Source: CAD feature listing. Evaluate the final solid. Frame: model axes, mm. A direction names the side the tool comes from. Coordinates: 2 decimals unless noted, no trailing zeros. Loops run counter-clockwise (first coordinate to the right, second up) from the corner with the lowest first, then second, coordinate; pieces in that order, holes last.
Item 1: Section query A-A, the plane y = 0. Return the cut outline in (x, z), then the cut area to 3 significant figures.
Item 2: Section query B-B, the plane x = -79.5. Return the cut outline in (y, z).
Item 3: Pin query (flat end, axial travel): pin 1 Ø3 at (x, z) = (-99.5, 72.5) entering from +Y; pin 2 Ø8 at (y, z) = (-39.5, 93) entering from +X; pin 3 Ø6 at (x, z) = (-19.5, 170) entering from +Y. Return the tip coordinate at first contact, or that it passes through.
Item 4: Section query D-D, the plane y = 279. Return the cut outline in (x, z).
Item 5: Line query: probe 1 along Y at (x, z) = (0, 71); probe 2 along Z at (x, y) = (103.5, 95.5); probe 3 along Z at (x, y) = (82, 193). Output: solid intervals per line, ascending.
Item 6: Reachability of faces 1 (the flat face through (100, 210, 188)), 2 (the cylindrical face through (-19.527, 148.724, -7.395)), 3 (the cylindrical face through (123.997, -39.048, 88.74)) from +Z, -Z, +X, -X, +Y, -Y: full face, straight path, thin tool, end or side. Return the list, or none.
Item 7: Pull-direction query (X, two-part tool) for faces 4 (the flat face through (1, 311.803, 188)), 5 (the flat face through (-100, 213, 188)), 6 (the cylindrical face through (-30.04, -95.38, 88.53)); classes: +X half, -X half, draft (parallel to the pull), parting line (faces both ways), or undercut.
Item 8: Section query C-C, the plane z = 68.5. Return the cut outline in (x, y).
Autodesk Inventor part; units mm, degrees
ref_plane "Work Plane3" through (0, 0, 90) normal (0, 0, -1) x (-1, 0, 0)
ref_plane "YZ Plane" through (0, 0, 0) normal (1, 0, 0) x (0, 1, 0)
ref_plane "XZ Plane" through (0, 0, 0) normal (0, 1, 0) x (-1, 0, 0)
sketch "Sketch1" plane through (0, 0, 0) normal (0, 0, 1) x (1, 0, 0)
  circle A0 centre (0, 0) radius 130
  dimension "d0" = 260
extrude "Extrusion1" add sketch "Sketch1" along normal blind 180
sketch "Sketch2" plane through (0, 0, 180) normal (0, 0, 1) x (1, 0, 0)
  circle A0 centre (0, 0) radius 150
  dimension "d3" = 300
extrude "Extrusion2" add sketch "Sketch2" along normal blind 15
ref_plane "Work Plane3" through (0, 0, 90) normal (0, 0, -1) x (-1, 0, 0)
mirror "Mirror2" about plane through (0, 0, 90) normal (0, 0, -1) of "Extrusion2"
hole "Hole2" at (0, 0, 195) direction (0, 0, -1) diameter 200 end through all
sketch "Sketch6" plane through (0, 0, 195) normal (0, 0, 1) x (1, 0, 0)
  line L0 (-100, 111.8034) -> (100, 111.8034) construction
  line L1 (100, 111.8034) -> (100, 311.8034)
  line L2 (100, 311.8034) -> (-100, 311.8034)
  line L3 (-100, 311.8034) -> (-100, 111.8034)
  circle A0 centre (0, 0) radius 150
  dimension "d36" = 200
  dimension "d37" = 200
extrude "Extrusion6" add sketch "Sketch6" against normal blind 15 contours A0 L3 L2 L1
properties part number "Generator placement"
Verdict:
1. outline: (-150, -15) - (-100, -15) - (-100, 195) - (-150, 195) - (-150, 180) - (-130, 180) - (-130, 0) - (-150, 0) - close; (100, -15) - (150, -15) - (150, 0) - (130, 0) - (130, 180) - (150, 180) - (150, 195) - (100, 195) - close
1. area: 13,800 mm2
2. outline: (-127.2, -15) - (-60.66, -15) - (-60.66, 195) - (-127.2, 195) - (-127.2, 180) - (-102.86, 180) - (-102.86, 0) - (-127.2, 0) - close; (60.66, -15) - (127.2, -15) - (127.2, 0) - (102.86, 0) - (102.86, 180) - (311.8, 180) - (311.8, 195) - (60.66, 195) - close
3. pin 1: stops at y = 85.42
3. pin 2: stops at x = 125.06
3. pin 3: stops at y = 128.95
4. outline: (-100, 180) - (100, 180) - (100, 195) - (-100, 195) - close
5. probe 1: y = -130 to -100, 100 to 130
5. probe 2: z = -15 to 0, 180 to 195
5. probe 3: z = 180 to 195
6. face 1: +Z, -Z, +X, +Y
6. face 2: -Z
6. face 3: none
7. face 4: draft
7. face 5: -X half
7. face 6: undercut
8. outline: circle Ø260 at (0, 0); hole circle Ø200 at (0, 0)
